Source: CAD feature listing. Evaluate the final solid. Frame: model axes, mm. A direction names the side the tool comes from. Give positions to 0.01 mm unless a question says otherwise; leave off trailing zeros. Loops run counter-clockwise (first coordinate to the right, second up) from the corner with the lowest first, then second, coordinate; pieces in that order, holes last. Notation, with made-up numbers: (-18, -26.75) -> (41, -26.75) arc R23 ccw to (41, 10.25) -> close; hole circle Ø5 at (35, 76). An arc over 180 degrees is marked (long way). Return JSON: item names as keys, results as strings. Group by question number.
(1) Access query for faces 1 (the face through (3.24, 2.33, 2.03)), 2 (the face through (5.07, 0.285, 6.199)). Directions: +Z, -Z, +X, -X, +Y, -Y. A direction counts if a zero-diameter tool reaches every point of the face in a straight line with its end or side. Return the directions, or none.
(2) Cut plane A-A on z = 3.25. Return loops of the section in (x, y), then the cut area to 3 significant figures.
(3) Ray query, line 1 (X direction, y = 3.5, z = 1.5); line 2 (X direction, y = 2.5, z = 3). Return the intervals inside material, ascending. Write a range as from..to.
(4) Cut plane C-C on z = 6.25. Return loops of the section in (x, y).
(5) Cut plane B-B on y = 0.5. Return loops of the section in (x, z).
(6) Draft query along X for faces 3 (the face through (0, 5, 3)), 4 (the face through (3.388, 3.676, 4.596)), 5 (the face through (4.563, 9.715, 6.199)). Return one class per face: released by +X, released by -X, zero draft, split by the parting line, or undercut.
```python
from build123d import *

# Parameters (mm, degrees)
SKETCH1_W                = 10
SKETCH1_H                = 10
BOSS_EXTRUDE1_DEPTH      = 6.5
FILLET1_R                = 1
M2_CLEARANCE_HOLE1_D     = 2.4
M2_CLEARANCE_HOLE1_DEPTH = 4
M2_CLEARANCE_HOLE1_TIP   = 0.721032743


with BuildPart() as part:
    # Sketch1 → Boss-Extrude1 (new body)
    with BuildSketch(Plane.XY):
        with Locations((5, 5)):
            Rectangle(SKETCH1_W, SKETCH1_H)
    extrude(amount=BOSS_EXTRUDE1_DEPTH)

    # Fillet1
    fillet1_edges = [part.edges().sort_by_distance(p)[0] for p in [
        (10, 5, 6.5),
        (5, 10, 6.5),
        (0, 5, 6.5),
        (5, 0, 6.5),
        (10, 10, 3.25),
    ]]
    fillet(fillet1_edges, radius=FILLET1_R)

    # M2 Clearance Hole1
    with Locations(Plane(origin=(0, 0, 0), x_dir=(-1, 0, 0), z_dir=(0, 0, -1))):
        with Locations((-3.5, 3.5)):
            Hole(M2_CLEARANCE_HOLE1_D / 2, depth=M2_CLEARANCE_HOLE1_DEPTH)
            with Locations((0, 0, -(M2_CLEARANCE_HOLE1_DEPTH + M2_CLEARANCE_HOLE1_TIP / 2))):  # 118° drill point
                Cone(0, M2_CLEARANCE_HOLE1_D / 2, M2_CLEARANCE_HOLE1_TIP, mode=Mode.SUBTRACT)


solid = part.part
```
Answers:
{
 "1": {"face 1": "-Z", "face 2": "+Z, +X, -X, -Y"},
 "2": {"outline": "(0, 0) -> (10, 0) -> (10, 9) arc R1 ccw to (9, 10) -> (0, 10) -> close; hole circle Ø2.4 at (3.5, 3.5)", "area": "95.3 mm²"},
 "3": {"line 1": "0..2.3, 4.7..10", "line 2": "0..2.84, 4.16..10"},
 "4": {"outline": "(0.34, 0.34) -> (9.66, 0.34) -> (9.66, 9) arc R0.66 ccw to (9, 9.66) -> (0.34, 9.66) -> close"},
 "5": {"outline": "(0, 0) -> (10, 0) -> (10, 5.5) arc R1 ccw to (9.5, 6.37) -> (0.5, 6.37) arc R1 ccw to (0, 5.5) -> close"},
 "6": {"face 3": "released by -X", "face 4": "undercut", "face 5": "zero draft"}
}
